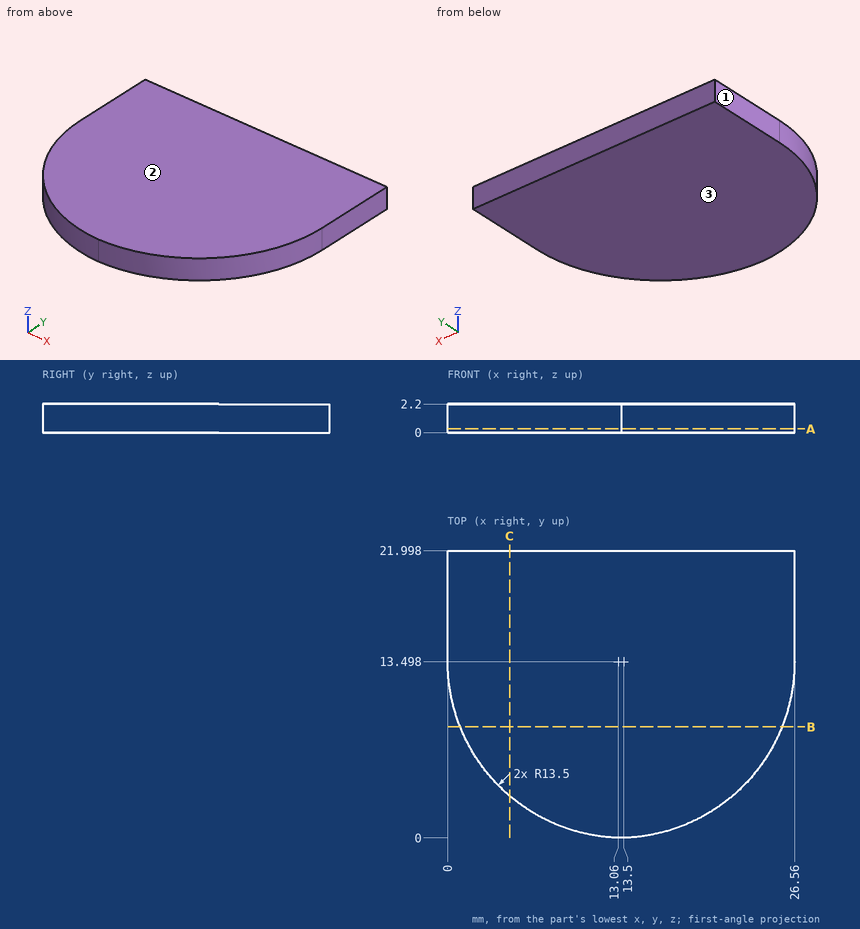
Drawing for the job (mm, zero at the part's lowest x, y, z). Give positions to 0.01 mm unless a question says otherwise; leave off trailing zeros. Loops run counter-clockwise (first coordinate to the right, second up) from the corner with the lowest first, then second, coordinate; pieces in that order, holes last.
(1) Band-saw the part on C-C (x = 4.75). Write the cut outline in (y, z), and give its area (3 significant figures).
Return value:
outline: (3.22, 0) - (22, 0) - (22, 2.2) - (3.22, 2.2) - close
area: 41.3 mm2
(2) Pin check, flat tips, straight feed: pin 1 (1 mm diameter, centred on y = 3, z = 1, fed in from -X); pin 2 (1 mm diameter, centred on x = 15, z = 1.5, fed in from -Y) (1 decimal); pin 3 (1 mm diameter, centred on y = 9, z = 0.5, fed in from -X). Stop position of each tip, or through.
Return value:
pin 1: stops at x = 4.43
pin 2: stops at y = 0.1
pin 3: stops at x = 0.61
(3) Band-saw the part on B-B (y = 8.5). Write the cut outline in (x, z).
Return value:
outline: (0.96, 0) - (25.6, 0) - (25.6, 2.2) - (0.96, 2.2) - close
(4) Band-saw the part on A-A (z = 0.3). Write the cut outline in (x, y), and give its area (3 significant figures).
Return value:
outline: (0, 13.5) arc R13.5 ccw to (13.28, 0) arc R13.5 ccw to (26.56, 13.5) - (26.56, 22) - (0, 22) - close
area: 506 mm2
(5) Pull direction Z, two halves, no side cores. Call the marked faces 1, 2 and 3: pulls with the +Z half, pulls with the -Z half, needs draft (parallel to the pull), parting line crosses it, or undercut.
Return value:
face 1: needs draft
face 2: pulls with the +Z half
face 3: pulls with the -Z half
(6) Drill centre lines: line 1 along Y through (x, z) = (11.5, 2); line 2 along Y through (x, z) = (19, 0.6) (1 decimal); line 3 along X through (y, z) = (2.25, 1.5) (1 decimal). Where is each one in solid material? Low to high.
Return value:
line 1: y = 0.15 to 22
line 2: y = 1.4 to 22
line 3: x = 6 to 20.5
